Geometry check sheet. Reference: drawing and pictorial views, mm from the part's lowest x, y, z. Round coordinates to 2 decimals unless told otherwise and drop trailing zeros. Order: outer loops, then holes, each group sorted by start corner. A loop starts at its lowest first (then second) coordinate and runs counter-clockwise, first axis right, second up.
(1) Sectioned sample at C-C (x = 4). Record the boundary of the cut face in (y, z), plus the area to 3 significant figures.
(2) Sectioned sample at D-D (z = 8.5). Record the boundary of the cut face in (x, y), plus the area to 3 significant figures.
(3) Go/stop test with flat-tipped pins: pin 1 (5 mm diameter, centred on x = 23, z = 7, fed in from -Y); pin 2 (5.5 mm diameter, centred on y = 122, z = 1.5, fed in from -X); pin 3 (5.5 mm diameter, centred on y = 86.5, z = 3.5, fed in from +X); pin 4 (3 mm diameter, centred on y = 136, z = 8.5, fed in from -X). Record where each tip stops, or that it passes through.
(4) Release check for a two-part mould opening along Y. For the marked faces 1 and 2 record: +Y half, -Y half, draft (parallel to the pull), parting line (faces both ways), or undercut.
(5) Sectioned sample at A-A (x = 19.05). Record the boundary of the cut face in (y, z).
(6) Material ranges on line 1 along Y through (x, z) = (19, 6); line 2 along Z through (x, y) = (36.5, 26.5); line 3 along Y through (x, z) = (5, 2.5) (1 decimal), recorded low to high.
(7) Sectioned sample at B-B (y = 19.05). Record the boundary of the cut face in (x, z), plus the area to 3 significant figures.
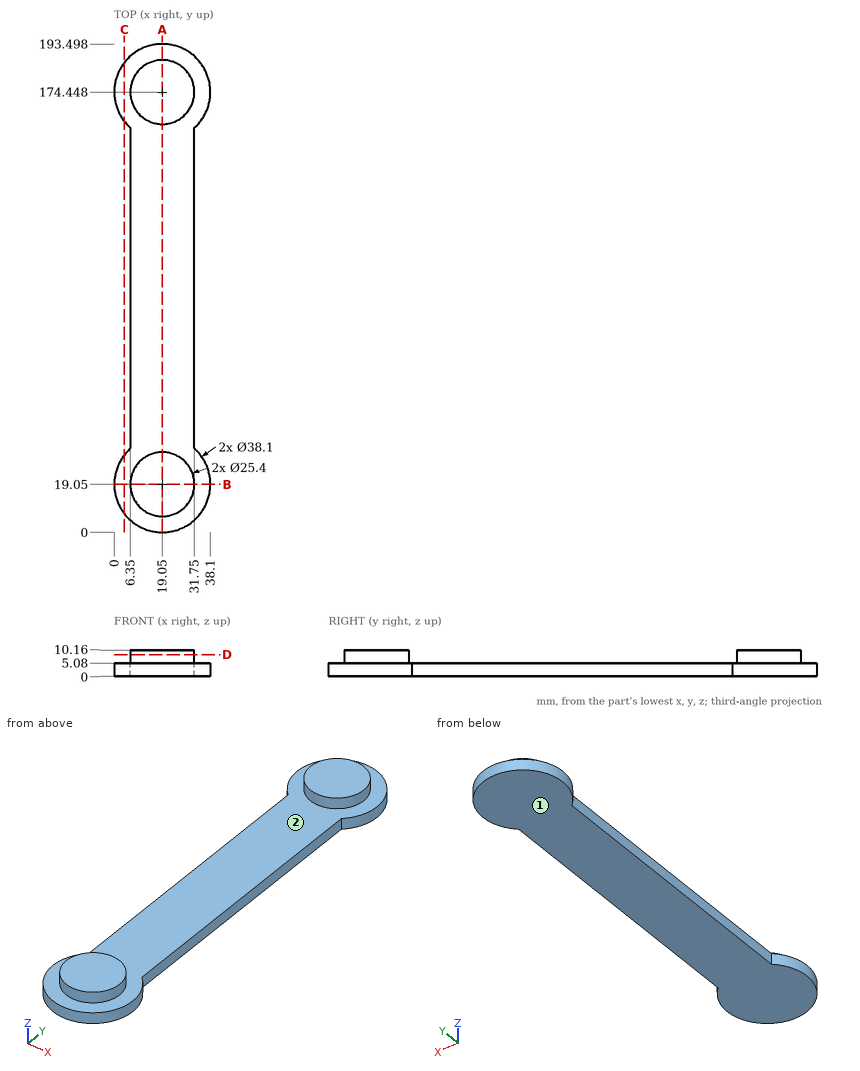
Answer below:
1. outline: (7.37, 0) - (30.73, 0) - (30.73, 5.08) - (7.37, 5.08) - close; (162.77, 0) - (186.13, 0) - (186.13, 5.08) - (162.77, 5.08) - close
1. area: 237 mm2
2. outline: circle Ø25.4 at (19.05, 19.05); circle Ø25.4 at (19.05, 174.45)
2. area: 1,010 mm2
3. pin 1: stops at y = 0.15
3. pin 2: stops at x = 6.35
3. pin 3: stops at x = 31.75
3. pin 4: passes through
4. face 1: draft
4. face 2: undercut
5. outline: (0, 0) - (193.5, 0) - (193.5, 5.08) - (187.15, 5.08) - (187.15, 10.16) - (161.75, 10.16) - (161.75, 5.08) - (31.75, 5.08) - (31.75, 10.16) - (6.35, 10.16) - (6.35, 5.08) - (0, 5.08) - close
6. line 1: y = 6.35 to 31.75, 161.75 to 187.15
6. line 2: z = 0 to 5.08
6. line 3: y = 6.2 to 31.9, 161.6 to 187.3
7. outline: (0, 0) - (38.1, 0) - (38.1, 5.08) - (31.75, 5.08) - (31.75, 10.16) - (6.35, 10.16) - (6.35, 5.08) - (0, 5.08) - close
7. area: 323 mm2
